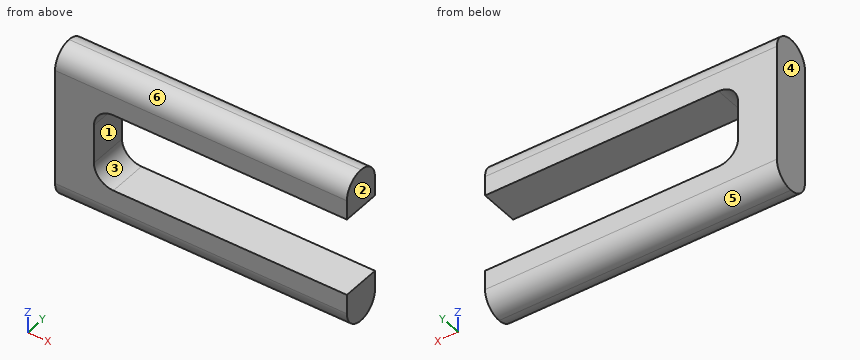
from build123d import *

# Parameters (mm, degrees)
F1_DEPTH = 2
F2_R     = 1.99999


# Not quite as in the source:
# - a fillet or chamfer is up to 0.001 mm smaller than in the source, because OpenCascade refuses the exact size


with BuildPart() as f1:
    # F0 (on Front) → F1 (new body, symmetric)
    with BuildSketch(Plane.XZ):
        Polygon((0, 12), (0, 16), (-30, 16), (-30, 0), (0, 0), (0, 4), (-26, 4), (-26, 12), align=None)
    extrude(amount=F1_DEPTH, both=True)

    # F2 (radius 2 in the source; OpenCascade refuses exactly that, so slightly less here)
    f2_edges = [f1.edges().sort_by_distance(p)[0] for p in [
        (-15, -2, 16),
        (-15, 2, 16),
        (-15, -2, 0),
        (-15, 2, 0),
        (-26, 0, 4),
        (-26, 0, 12),
    ]]
    fillet(f2_edges, radius=F2_R)


solid = f1.part
The model under review builds one solid part; all positions refer to its coordinate system, in mm. Face numbers are marked on the shaded views. A direction names the side the tool comes from. Round coordinates to 2 decimals unless told otherwise and drop trailing zeros. Loops run counter-clockwise (first coordinate to the right, second up) from the corner with the lowest first, then second, coordinate; pieces in that order, holes last. Notation, with made-up numbers: M 25.5,-39.5 L 42.5,-39.5 A22 cw 42.5,-24.5 Z; hole C 7,64 d4. An arc over 180 degrees is marked long. Answer as a JSON object with one key per item and string values.
Item 1: The part is to be moulded in two halves that separate along Z. For the marked faces 3, 4, 5 and 6, say which applies: +Z half, -Z half, draft (parallel to the pull), parting line (faces both ways), or undercut.
Check sheet entries:
{"face 3": "undercut", "face 4": "draft", "face 5": "-Z half", "face 6": "+Z half"}
Item 2: For line 1 along X through (y, z) = (0.65, 8.5); line 2 along Z through (x, y) = (-24.25, 1.7); line 3 along Z through (x, y) = (-4.5, -1.15), list the stretches that pass through material, from the lowest coordinate up.
Check sheet entries:
{"line 1": "-30 to -26", "line 2": "0.95 to 4.02, 11.98 to 15.05", "line 3": "0.36 to 4, 12 to 15.64"}
Item 3: Tool access review of the marked faces 1 and 2: name each direction out of +Z, -Z, +X, -X, +Y, -Y from which nothing blocks a thin tool from reaching the whole face with its end or side.
Check sheet entries:
{"face 1": "+X, +Y, -Y", "face 2": "+Z, -Z, +X, +Y, -Y"}
Item 4: We need section D-D, the plane z = 6.75. State the section outline as (x, y) points, and give its area (3 significant figures).
Check sheet entries:
{"outline": "M -30,-2 L -26,-2 L -26,2 L -30,2 Z", "area": "16.0 mm2"}
Item 5: We need section C-C, the plane y = 1.2. State the section outline as (x, z) points.
Check sheet entries:
{"outline": "M -30,0.4 L 0,0.4 L 0,4 L -24,4 A2 cw -26,6 L -26,10 A2 cw -24,12 L 0,12 L 0,15.6 L -30,15.6 Z"}
Item 6: Clearance check with flat-ended pins moving along their axes: P1, Ø1.2, axis at y = 0, z = 8.5, coming from the +X side; P2, Ø2, axis at y = -1, z = 3, coming from the +X side. State where each tip first meets the part, or that it passes through.
Check sheet entries:
{"P1": "x = -26", "P2": "x = 0"}
